Autodesk Fusion 360 part; units mm, degrees
sketch "Sketch1" plane through (0, 0, 0) normal (0, 1, 0) x (1, 0, 0)
  line L0 (-35, 18) -> (-29, 18)
  line L1 (-29, 18) -> (-29, 12)
  line L2 (-29, 12) -> (-35, 12)
  line L3 (-35, 12) -> (-35, 18)
sketch "Sketch2" plane through (0, 5, 0) normal (0, 1, 0) x (-1, 0, 0)
  line L0 (35, -12) -> (29, -12)
  line L1 (29, -12) -> (29, -18)
  line L2 (29, -18) -> (35, -18)
  line L3 (35, -18) -> (35, -12)
  line L4 (30, 0) -> (40, 0)
  line L5 (40, 0) -> (40, -10)
  line L6 (40, -10) -> (30, -10)
  line L7 (30, -10) -> (30, 0)
extrude "Extrude2" add sketch "Sketch2" along normal blind 10 contours L4 L5 L6 L7 makes body 1
sketch "Sketch3" plane through (0, 15, 0) normal (0, 1, 0) x (-1, 0, 0)
  line L0 (30, -10) -> (40, -10)
  line L1 (40, -10) -> (40, 0)
  line L2 (40, 0) -> (30, 0)
  line L3 (30, 0) -> (30, -10)
  line L4 (39.5, -9.5) -> (30.5, -9.5)
  line L5 (30.5, -9.5) -> (30.5, -0.5)
  line L6 (30.5, -0.5) -> (39.5, -0.5)
  line L7 (39.5, -0.5) -> (39.5, -9.5)
extrude "Extrude3" cut sketch "Sketch3" against normal blind 18 contours L4 L5 L6 L7 bodies 1
sketch "Sketch4" plane through (-30, 0, 0) normal (1, 0, 0) x (0, 0, -1)
  line L0 (0, 5) -> (10, 5)
  line L1 (10, 5) -> (10, 15)
  line L2 (10, 15) -> (0, 15)
  line L3 (0, 15) -> (0, 5)
  line L4 (0.5, 14.5) -> (9.5, 14.5)
  line L5 (9.5, 14.5) -> (9.5, 5.5)
  line L6 (9.5, 5.5) -> (0.5, 5.5)
  line L7 (0.5, 5.5) -> (0.5, 14.5)
  line L8 (0.5, 15) -> (0.5, 5)
  line L9 (9.5, 15) -> (9.5, 5)
extrude "Extrude4" cut sketch "Sketch4" against normal blind 16 contours L4 L5 L6 L7 L8 L9 bodies 1
sketch "Sketch5" plane through (0, 0, 0) normal (0, 0, 1) x (1, 0, 0)
  line L0 (-40, 5) -> (-30, 5)
  line L1 (-30, 5) -> (-30, 15)
  line L2 (-30, 15) -> (-40, 15)
  line L3 (-40, 15) -> (-40, 5)
  line L4 (-39.5, 14.5) -> (-30.5, 14.5)
  line L5 (-30.5, 14.5) -> (-30.5, 6)
  line L6 (-30.5, 6) -> (-39.5, 6)
  line L7 (-39.5, 6) -> (-39.5, 14.5)
  dimension "d9" = 8.5
extrude "Extrude5" cut sketch "Sketch5" against normal blind 23 contours L4 L5 L6 L7 bodies 1
sketch "Sketch6" plane through (0, 0, -10) normal (0, 0, -1) x (-1, 0, 0)
  line L0 (30.5, 6) -> (30.5, 14.5)
  line L1 (30.5, 14.5) -> (39.5, 14.5)
  line L2 (39.5, 14.5) -> (39.5, 6)
  line L3 (39.5, 6) -> (30.5, 6)
  line L4 (30, 5) -> (40, 5)
  line L5 (40, 5) -> (40, 15)
  line L6 (40, 15) -> (30, 15)
  line L7 (30, 15) -> (30, 5)
  line L8 (30.5, 6) -> (39.5, 6)
  line L9 (39.5, 6) -> (39.5, 5.5)
  line L10 (39.5, 5.5) -> (30.5, 5.5)
  line L11 (30.5, 5.5) -> (30.5, 6)
  point P0 (39.5, 5.5)
extrude "Extrude6" cut sketch "Sketch6" against normal blind 26.5 contours L3 L8 L9 L10 L11 bodies 1
sketch "Sketch7" plane through (0, 0, 0) normal (1, 0, 0) x (0, 0, -1)
sketch "Sketch8" plane through (0, 0, 0) normal (1, 0, 0) x (0, 0, -1)
  circle A0 centre (5, 10) radius 4.5568
  dimension "d15" = 9.1136
extrude "Extrude7" add sketch "Sketch8" along normal blind 10 separate body makes body 2
move_body "Move1" bodies 2 to x (1, 0, 0) y (0, 1, 0) z (0, 0, 1) at (-40, 0, 2)
move_body "Move2" bodies 2 to x (1, 0, 0) y (0, 1, 0) z (0, 0, 1) at (0, 0, -2)
sketch "Sketch9" plane through (-30, 0, 0) normal (1, 0, 0) x (0, 0, -1)
  circle A0 centre (5, 10) radius 4.5568
  circle A1 centre (5, 10) radius 4
  dimension "d24" = 8
extrude "Extrude8" cut sketch "Sketch9" against normal blind 18 contours A1 bodies 2
sketch "Sketch10" plane through (0, 0, 0) normal (0, 0, 1) x (1, 0, 0)
  circle A0 centre (-35.0032, 9.983) radius 4.5
  dimension "d27" = 9
extrude "Extrude9" cut sketch "Sketch10" against normal blind 22 bodies 1 2
combine "Combine1" operation add target body 1 tool bodies 2
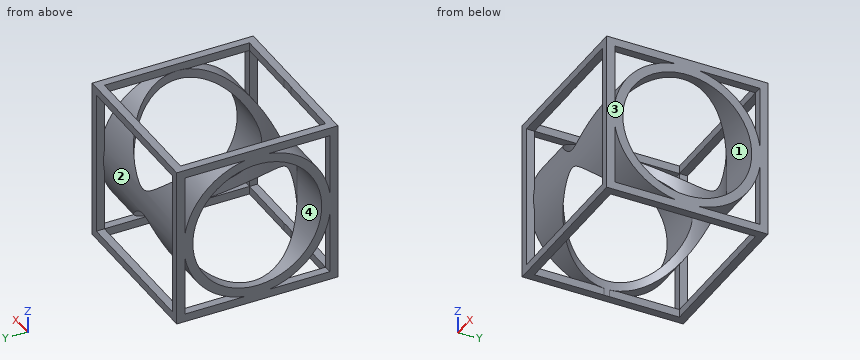
Input: part model. Units: mm. Frame: model coordinates. Face numbers are marked on the shaded views. A direction names the side the tool comes from. Round coordinates to 2 decimals unless told otherwise and drop trailing zeros. Loops run counter-clockwise (first coordinate to the right, second up) from the corner with the lowest first, then second, coordinate; pieces in that order, holes last. Notation, with made-up numbers: M 50.25,35 L 54.25,35 A21 ccw 54.25,51 Z; hole C -25,-31.75 d7. An arc over 180 degrees is marked long. Answer as CSV lines item,"result". Start each with the question number.
(1) Draft query along Y for the marked faces 3 and 4. Return one class per face: released by +Y, released by -Y, zero draft, split by the parting line, or undercut.
(2) Section D-D, the plane z = -5. Output: boundary loops of the cut face in (x, y).
(3) Section A-A, the plane x = -32. Output: boundary loops of the cut face in (y, z).
(4) Line query: line 1 (Y direction, x = -38.8, z = -5); line 2 (X direction, y = 14, z = -4.5); line 3 (Z direction, x = -38.5, y = 6.75). Output: solid intervals per line, ascending. Write a range as [from, to].
(5) Reachability of the marked faces 1 and 2 from +Z, -Z, +X, -X, +Y, -Y: full face, straight path, thin tool, end or side. Return the list, or none.
(6) Section B-B, the plane y = 11.25. State how many separate pieces and enclosed holes the cut face has, plus the area to 3 significant figures.
Values found:
1,face 3,"zero draft"
1,face 4,"undercut"
2,outline,"M -40,5 L -39.5,5 L -39.5,5.44 L -30.5,5.44 L -30.5,5 L -30,5 L -30,6 L -32.91,6 A4.5 cw -37.1,6 L -40,6 Z; M -40,14 L -37.03,14 A4.5 cw -32.97,14 L -30,14 L -30,15 L -30.5,15 L -30.5,14.56 L -39.5,14.56 L -39.5,15 L -40,15 Z"
3,outline,"M 5,-10 L 5.5,-10 L 5.5,-9.5 L 5,-9.5 Z; M 5,-0.5 L 5.5,-0.5 L 5.5,0 L 5,0 Z; M 6.63,-8.07 L 6.63,-7.16 A4 cw 6.63,-2.84 L 6.63,-1.93 A4.56 ccw Z; M 13.33,-8.11 A4.56 ccw 13.33,-1.89 L 13.33,-2.79 A4 cw 13.33,-7.21 Z; M 14.5,-10 L 15,-10 L 15,-9.5 L 14.5,-9.5 Z; M 14.5,-0.5 L 15,-0.5 L 15,0 L 14.5,0 Z"
4,line 1,"y = [5.44, 6], [14, 14.56]"
4,line 2,"x = [-40, -37.03], [-32.97, -30]"
4,line 3,"z = [-8.19, -7.33], [-2.67, -1.81]"
5,face 1,"+X, -X"
5,face 2,"none"
6,separate pieces,"8"
6,enclosed holes,"0"
6,area,"2.59 mm²"
